Check sheet for the modelled part. Datum: model origin and axes. Units: mm. Give positions to 0.01 mm unless a question says otherwise; leave off trailing zeros. Loops run counter-clockwise (first coordinate to the right, second up) from the corner with the lowest first, then second, coordinate; pieces in that order, holes last. Notation, with made-up numbers: M 64.25,1.5 L 84.25,1.5 A26 ccw 84.25,37.5 Z; hole C 59.5,69.25 d8. An arc over 180 degrees is marked long. Use one line per item in the form item = value.
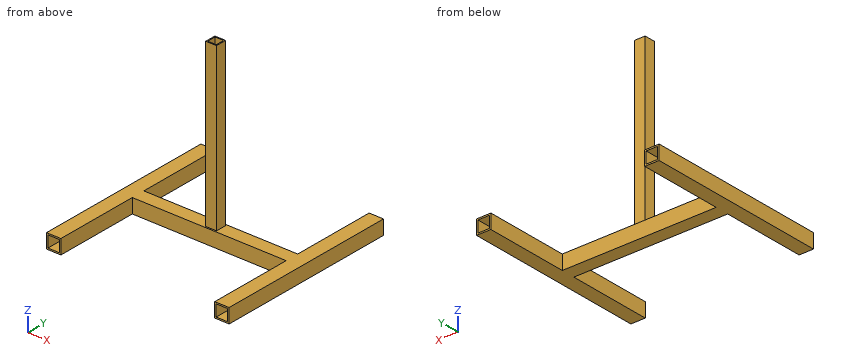
from build123d import *

# Parameters (mm, degrees)
F0_W     = 40
F0_H     = 40
F0_W_2   = 32
F0_H_2   = 32
F1_DEPTH = 508
F2_W     = 38.1
F2_H     = 40
F2_W_2   = 25.4
F2_H_2   = 27.3
F3_DEPTH = 431.8
F4_W     = 30
F4_H     = 30
F4_W_2   = 24
F4_H_2   = 24
F5_DEPTH = 450


with BuildPart() as f1:
    # F0 (on Front) → F1 (new body)
    with BuildSketch(Plane.XZ):
        with Locations((-234, 20)):
            Rectangle(F0_W, F0_H)
        with Locations((-234, 20)):
            Rectangle(F0_W_2, F0_H_2, mode=Mode.SUBTRACT)
    extrude(amount=-F1_DEPTH)



with BuildPart() as f1b:
    # F0 (on Front) → F1, piece 2 (new body)
    with BuildSketch(Plane.XZ):
        with Locations((234, 20)):
            Rectangle(F0_W, F0_H)
        with Locations((234, 20)):
            Rectangle(F0_W_2, F0_H_2, mode=Mode.SUBTRACT)
    extrude(amount=-F1_DEPTH)


with BuildPart() as f1_1:
    add(f1.part)

    add(f1b.part)  # F3 merges F1b
    # F2 (on face) → F3 (join)
    with BuildSketch(Plane.YZ.offset(-214)):
        with Locations((254, 20)):
            Rectangle(F2_W, F2_H)
        with Locations((254, 20)):
            Rectangle(F2_W_2, F2_H_2, mode=Mode.SUBTRACT)
    extrude(amount=F3_DEPTH)

    # F4 (on face) → F5 (join)
    with BuildSketch(Plane.XY.offset(40)):
        with Locations((1.9, 254)):
            Rectangle(F4_W, F4_H)
        with Locations((1.9, 254)):
            Rectangle(F4_W_2, F4_H_2, mode=Mode.SUBTRACT)
    extrude(amount=F5_DEPTH)


solid = f1_1.part
1) Section check C-C (z = 384.5). Record the cut outline in (x, y).
Evaluation:
outline = M -13.1,239 L 16.9,239 L 16.9,269 L -13.1,269 Z; hole M -10.1,242 L 13.9,242 L 13.9,266 L -10.1,266 Z
2) Scan lines: line 1 (Z direction, x = -230.5, y = 327); line 2 (Z direction, x = 93.5, y = 264.5); line 3 (X direction, y = 149.5, z = 39). Record each from-to range of solid material in increasing order.
Evaluation:
line_1 = 0 to 4, 36 to 40
line_2 = 0 to 6.35, 33.65 to 40
line_3 = -254 to -214, 214 to 254
3) Section check A-A (y = 420.5). Record the cut outline in (x, z), then the cut area to 3 significant figures.
Evaluation:
outline = M -254,0 L -214,0 L -214,40 L -254,40 Z; M 214,0 L 254,0 L 254,40 L 214,40 Z; hole M -250,4 L -218,4 L -218,36 L -250,36 Z; hole M 218,4 L 250,4 L 250,36 L 218,36 Z
area = 1,150 mm^2
4) Section check B-B (x = 187). Record the cut outline in (y, z), then the cut area to 3 significant figures.
Evaluation:
outline = M 234.95,0 L 273.05,0 L 273.05,40 L 234.95,40 Z; hole M 241.3,6.35 L 266.7,6.35 L 266.7,33.65 L 241.3,33.65 Z
area = 831 mm^2
5) Depth check by flat-ended pin: pin 1 Ø12 at (x, z) = (54.5, 11) entering from -Y; pin 2 Ø12 at (x, z) = (20, 20) entering from +Y; pin 3 Ø10 at (y, z) = (244, 157) entering from +X. Enter the tip coordinate at first touch or a pass-through.
Evaluation:
pin_1 = 234.95
pin_2 = 273.05
pin_3 = 16.9
